Can you work these out from the model? Positions are in its coordinate system, mm. A direction names the side the tool comes from. Round coordinates to 2 decimals unless told otherwise and drop trailing zeros. Write each loop counter-clockwise with the first axis right and the second up, starting at its lowest first coordinate (ties: lowest second). Pieces come first, ordered by that corner, then holes. Notation, with made-up numbers: (30.25, 24.25) -> (78.25, 24.25) arc R37 cw to (78.25, 63.25) -> close; hole circle Ø7 at (40, 62.25). An arc over 180 degrees is marked (long way). Write item = value, one per line. Start each with the question number.
1) If I drill on line 1 (X direction, y = -23, z = -54); line 2 (Y direction, x = 86.5, z = -20.5); line 3 (Z direction, x = 66.5, y = 77.5), over which ranges is the centre line in solid material (lowest first)?
2) For faces 1 (the face through (-13, 194.34, -30)), 2 (the face through (-13, 60, 3)), which set-ups out of +Z, -Z, +X, -X, +Y, -Y let a thin tool reach every point of the face, with its end or its side?
3) I'm going to push a flat-ended pin straight in: pin 1 (7 mm diameter, centred on x = -90.61, y = -18.18, fed in from -Z). Where does the tip first touch, or does it pass through?
4) Imagine slicing it at A-A, the plane z = -17.5. Please give me the cut outline in (x, y), then the cut area to 3 significant figures.
5) Imagine slicing it at C-C, the plane y = 124.5. Please give me the cut outline in (x, z), then the cut area to 3 significant figures.
6) Imagine slicing it at B-B, the plane x = -98.5. Please give me the cut outline in (y, z).
7) Thinking about a two-plate mould opening in X: for faces 3 (the face through (-13, 197.34, -28)), 4 (the face through (93.902, 56, -30)), 5 (the face through (96.902, 56, -28)), which applies, +X half, -X half, draft (parallel to the pull), parting line (faces both ways), or undercut?
from build123d import *

# Parameters (mm, degrees)
SKETCH1_W           = 215.9
SKETCH1_H           = 279.4
BOSS_EXTRUDE1_DEPTH = 3
SKETCH2_W           = 215.9
SKETCH2_H           = 279.4
SKETCH2_W_2         = 209.9
SKETCH2_H_2         = 273.4
BOSS_EXTRUDE2_DEPTH = 63.5
SKETCH3_R           = 3
SKETCH3_R_2         = 3.05
CUT_EXTRUDE3_DEPTH  = 5


with BuildPart() as part:
    # Sketch1 → Boss-Extrude1 (new body)
    with BuildSketch(Plane.XY):
        with Locations((-11.047990366, 57.640345361)):
            Rectangle(SKETCH1_W, SKETCH1_H)
    extrude(amount=BOSS_EXTRUDE1_DEPTH)

    # Sketch2 → Boss-Extrude2 (add)
    with BuildSketch(Plane.XY.offset(3)):
        with Locations((-11.047990366, 57.640345361)):
            Rectangle(SKETCH2_W, SKETCH2_H)
        with Locations((-11.047990366, 57.640345361)):
            Rectangle(SKETCH2_W_2, SKETCH2_H_2, mode=Mode.SUBTRACT)
    extrude(amount=-BOSS_EXTRUDE2_DEPTH)

    # Sketch3 → Cut-Extrude3 (cut)
    with BuildSketch(Plane(origin=(0, 0, 0), x_dir=(-1, 0, 0), z_dir=(0, 0, -1))):
        with Locations((-68.517009634, -18.179654639)):
            Circle(SKETCH3_R)
        with Locations((-72.517009634, 92.080345361)):
            Circle(SKETCH3_R)
        with Locations((-38.517009634, 184.340345361)):
            Circle(SKETCH3_R)
        with Locations((90.612990366, 92.080345361)):
            Circle(SKETCH3_R)
        with Locations((-58.712009634, -93.094201664)):
            Circle(SKETCH3_R)
        with Locations((90.612990366, 184.340345361)):
            Circle(SKETCH3_R)
        with Locations((90.612990366, -18.179654639)):
            Circle(SKETCH3_R_2)
    extrude(amount=-CUT_EXTRUDE3_DEPTH, mode=Mode.SUBTRACT)


solid = part.part
Reported:
q1.line_1 = -119 to -116, 93.9 to 96.9
q1.line_2 = -82.06 to -79.06, 194.34 to 197.34
q1.line_3 = 0 to 3
q2.face_1 = -Z
q2.face_2 = +Z, +X, -X, +Y, -Y
q3.pin_1 = 0
q4.outline = (-119, -82.06) -> (96.9, -82.06) -> (96.9, 197.34) -> (-119, 197.34) -> close; hole (-116, -79.06) -> (93.9, -79.06) -> (93.9, 194.34) -> (-116, 194.34) -> close
q4.area = 2,940 mm²
q5.outline = (-119, -60.5) -> (-116, -60.5) -> (-116, 0) -> (93.9, 0) -> (93.9, -60.5) -> (96.9, -60.5) -> (96.9, 3) -> (-119, 3) -> close
q5.area = 1,010 mm²
q6.outline = (-82.06, -60.5) -> (-79.06, -60.5) -> (-79.06, 0) -> (194.34, 0) -> (194.34, -60.5) -> (197.34, -60.5) -> (197.34, 3) -> (-82.06, 3) -> close
q7.face_3 = draft
q7.face_4 = undercut
q7.face_5 = +X half
